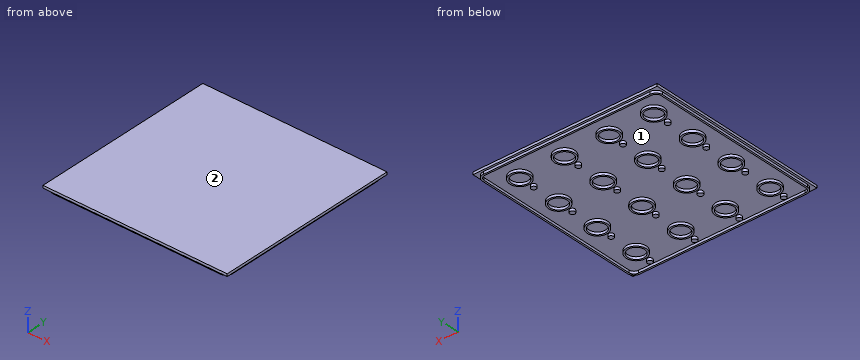
from build123d import *

# Parameters (mm, degrees)
SKETCH_W      = 110
SKETCH_H      = 110
PAD_DEPTH     = 1.5
PAD001_DEPTH  = 1.5
SKETCH002_R   = 6
SKETCH002_R_2 = 5
SKETCH002_R_3 = 1.5
PAD002_DEPTH  = 1.5


with BuildPart() as part:
    # Sketch → Pad (new body)
    with BuildSketch(Plane.XY):
        Rectangle(SKETCH_W, SKETCH_H)
    extrude(amount=PAD_DEPTH)

    # Sketch001 → Pad001 (join)
    with BuildSketch(Plane(origin=(0, 0, 0), x_dir=(1, 0, 0), z_dir=(0, 0, -1))):
        with BuildLine():
            Line((-49.8, 53.8), (49.8, 53.8))
            ThreePointArc((53.8, 49.8), (52.628427, 52.628427), (49.8, 53.8))
            Line((53.8, 49.8), (53.8, -49.8))
            ThreePointArc((49.8, -53.8), (52.628427, -52.628427), (53.8, -49.8))
            Line((49.8, -53.8), (-49.8, -53.8))
            ThreePointArc((-53.8, -49.8), (-52.628427, -52.628427), (-49.8, -53.8))
            Line((-53.8, -49.8), (-53.8, 49.8))
            ThreePointArc((-49.8, 53.8), (-52.628427, 52.628427), (-53.8, 49.8))
        make_face()
        with BuildLine():
            Line((-49.8, 52.8), (49.8, 52.8))
            ThreePointArc((52.8, 49.8), (51.92132, 51.92132), (49.8, 52.8))
            Line((52.8, 49.8), (52.8, -49.8))
            ThreePointArc((49.8, -52.8), (51.92132, -51.92132), (52.8, -49.8))
            Line((49.8, -52.8), (-49.8, -52.8))
            ThreePointArc((-52.8, -49.8), (-51.92132, -51.92132), (-49.8, -52.8))
            Line((-52.8, -49.8), (-52.8, 49.8))
            ThreePointArc((-49.8, 52.8), (-51.92132, 51.92132), (-52.8, 49.8))
        make_face(mode=Mode.SUBTRACT)
    extrude(amount=PAD001_DEPTH)

    # Sketch002 → Pad002 (join)
    with BuildSketch(Plane(origin=(0, 0, 0), x_dir=(1, 0, 0), z_dir=(0, 0, -1))):
        with Locations((-40.005, 40.005)):
            Circle(SKETCH002_R)
        with Locations((-40.005, 40.005)):
            Circle(SKETCH002_R_2, mode=Mode.SUBTRACT)
        with Locations((-40.005, 49.505)):
            Circle(SKETCH002_R_3)
        with Locations((-13.335, 40.005)):
            Circle(SKETCH002_R)
        with Locations((-13.335, 40.005)):
            Circle(SKETCH002_R_2, mode=Mode.SUBTRACT)
        with Locations((-13.335, 49.505)):
            Circle(SKETCH002_R_3)
        with Locations((13.335, 40.005)):
            Circle(SKETCH002_R)
        with Locations((13.335, 40.005)):
            Circle(SKETCH002_R_2, mode=Mode.SUBTRACT)
        with Locations((13.335, 49.505)):
            Circle(SKETCH002_R_3)
        with Locations((40.005, 40.005)):
            Circle(SKETCH002_R)
        with Locations((40.005, 40.005)):
            Circle(SKETCH002_R_2, mode=Mode.SUBTRACT)
        with Locations((40.005, 49.505)):
            Circle(SKETCH002_R_3)
        with Locations((-40.005, 13.335)):
            Circle(SKETCH002_R)
        with Locations((-40.005, 13.335)):
            Circle(SKETCH002_R_2, mode=Mode.SUBTRACT)
        with Locations((-40.005, 22.835)):
            Circle(SKETCH002_R_3)
        with Locations((-13.335, 13.335)):
            Circle(SKETCH002_R)
        with Locations((-13.335, 13.335)):
            Circle(SKETCH002_R_2, mode=Mode.SUBTRACT)
        with Locations((-13.335, 22.835)):
            Circle(SKETCH002_R_3)
        with Locations((13.335, 13.335)):
            Circle(SKETCH002_R)
        with Locations((13.335, 13.335)):
            Circle(SKETCH002_R_2, mode=Mode.SUBTRACT)
        with Locations((13.335, 22.835)):
            Circle(SKETCH002_R_3)
        with Locations((40.005, 13.335)):
            Circle(SKETCH002_R)
        with Locations((40.005, 13.335)):
            Circle(SKETCH002_R_2, mode=Mode.SUBTRACT)
        with Locations((40.005, 22.835)):
            Circle(SKETCH002_R_3)
        with Locations((-40.005, -13.335)):
            Circle(SKETCH002_R)
        with Locations((-40.005, -13.335)):
            Circle(SKETCH002_R_2, mode=Mode.SUBTRACT)
        with Locations((-40.005, -3.835)):
            Circle(SKETCH002_R_3)
        with Locations((-13.335, -13.335)):
            Circle(SKETCH002_R)
        with Locations((-13.335, -13.335)):
            Circle(SKETCH002_R_2, mode=Mode.SUBTRACT)
        with Locations((-13.335, -3.835)):
            Circle(SKETCH002_R_3)
        with Locations((13.335, -13.335)):
            Circle(SKETCH002_R)
        with Locations((13.335, -13.335)):
            Circle(SKETCH002_R_2, mode=Mode.SUBTRACT)
        with Locations((13.335, -3.835)):
            Circle(SKETCH002_R_3)
        with Locations((40.005, -13.335)):
            Circle(SKETCH002_R)
        with Locations((40.005, -13.335)):
            Circle(SKETCH002_R_2, mode=Mode.SUBTRACT)
        with Locations((40.005, -3.835)):
            Circle(SKETCH002_R_3)
        with Locations((-40.005, -40.005)):
            Circle(SKETCH002_R)
        with Locations((-40.005, -40.005)):
            Circle(SKETCH002_R_2, mode=Mode.SUBTRACT)
        with Locations((-40.005, -30.505)):
            Circle(SKETCH002_R_3)
        with Locations((-13.335, -40.005)):
            Circle(SKETCH002_R)
        with Locations((-13.335, -40.005)):
            Circle(SKETCH002_R_2, mode=Mode.SUBTRACT)
        with Locations((-13.335, -30.505)):
            Circle(SKETCH002_R_3)
        with Locations((13.335, -40.005)):
            Circle(SKETCH002_R)
        with Locations((13.335, -40.005)):
            Circle(SKETCH002_R_2, mode=Mode.SUBTRACT)
        with Locations((13.335, -30.505)):
            Circle(SKETCH002_R_3)
        with Locations((40.005, -40.005)):
            Circle(SKETCH002_R)
        with Locations((40.005, -40.005)):
            Circle(SKETCH002_R_2, mode=Mode.SUBTRACT)
        with Locations((40.005, -30.505)):
            Circle(SKETCH002_R_3)
    extrude(amount=PAD002_DEPTH)


solid = part.part
Design review of the part built by this model. Coordinates are the model's own, in mm. Face numbers are marked on the shaded views. Round coordinates to 2 decimals unless told otherwise and drop trailing zeros. Write each loop counter-clockwise with the first axis right and the second up, starting at its lowest first coordinate (ties: lowest second). Pieces come first, ordered by that corner, then holes. Notation, with made-up numbers: (75, -19) - (84, -19) arc R19 cw to (84, -12) - close; hole circle Ø10 at (77.25, 16.5). An arc over 180 degrees is marked (long way). Use a Markdown table: item, result. Add a question column.
1. Clearance check with flat-ended pins moving along their axes: pin 1 (8 mm diameter, centred on x = 1, y = 0, fed in from -Z); pin 2 (0.8 mm diameter, centred on x = -1, z = -0.5, fed in from -Y); pin 3 (1.2 mm diameter, centred on y = -9, z = -1, fed in from +X); pin 4 (13 mm diameter, centred on x = -40.005, y = 13.335, fed in from -Z). State where each tip first meets the part, or that it passes through.
2. We need section A-A (x = -5.5). State the section outline as (y, z) points, then the cut area to 3 significant figures.
3. We need section B-B (z = -0.75). Count the separate pieces of the cut face and the enclosed holes in it, then the cut area to 3 significant figures.
4. Wall thickness on probe 1 along Y at (x, z) = (47.5, -1.25); probe 2 along Z at (x, y) = (-5, -0.5): over which ranges is each line inside the solid? List them lowest first.
5. Mouldability with a two-part tool opening along X and no side actions: class the marked faces 1 and 2 as +X half, -X half, draft (parallel to the pull), parting line (faces both ways), or undercut.
Output:
| question | item | result |
|---|---|---|
| 1 | pin 1 | stops at z = 0 |
| 1 | pin 2 | stops at y = -53.8 |
| 1 | pin 3 | stops at x = 53.8 |
| 1 | pin 4 | stops at z = -1.5 |
| 2 | outline | (-55, 0) - (-53.8, 0) - (-53.8, -1.5) - (-52.8, -1.5) - (-52.8, 0) - (52.8, 0) - (52.8, -1.5) - (53.8, -1.5) - (53.8, 0) - (55, 0) - (55, 1.5) - (-55, 1.5) - close |
| 2 | area | 168 mm2 |
| 3 | separate pieces | 33 |
| 3 | enclosed holes | 17 |
| 3 | area | 1,090 mm2 |
| 4 | probe 1 | y = -53.8 to -52.8, 52.8 to 53.8 |
| 4 | probe 2 | z = 0 to 1.5 |
| 5 | face 1 | undercut |
| 5 | face 2 | draft |
